Verification items for the finished model (mm, model axes). A direction names the side the tool comes from. Give positions to 0.01 mm unless a question says otherwise; leave off trailing zeros. Order: outer loops, then holes, each group sorted by start corner. A loop starts at its lowest first (then second) coordinate and runs counter-clockwise, first axis right, second up. Notation, with made-up numbers: (-9, 18) -> (41, 18) arc R14 cw to (41, 35) -> close; hole circle Ø4 at (-7, 34.5). An arc over 180 degrees is marked (long way). One line per question, with ' | ' between items. Start each with the question number.
Q1. Section check C-C on x = 52. Record the cut outline in (y, z).
Q2. Section check A-A on z = 5.25. Record the cut outline in (x, y) (1 decimal).
Q3. Go/stop test with flat-tipped pins: pin 1 (4 mm diameter, centred on x = -10.5, y = -47.5, fed in from -Z); pin 2 (1 mm diameter, centred on x = 41.5, z = 4, fed in from -Y); pin 3 (1.9 mm diameter, centred on x = -82, z = 4.5, fed in from +Y); pin 4 (2 mm diameter, centred on y = -67.5, z = 2, fed in from +X). Record where each tip stops, or that it passes through.
Q4. Material ranges on probe 1 along X at (y, z) = (52, 4.5); probe 2 along X at (y, z) = (76.5, 5.25) (3 decimals); probe 3 along Y at (x, z) = (29, 0.5), recorded low to high. Write a range as [from, to].
Q5. Section check B-B on y = 76.5. Record the cut outline in (x, z) (3 decimals), plus the area to 3 significant figures.
Q6. Mould release check, pull along Y, two halves, no side actions. Record for faces 3 (the cylindrical face through (-81.2, -79.6, 3.1)), 4 (the flat face through (9, 1, 0)): released by +Y, released by -Y, zero draft, split by the parting line, or undercut.
Q7. Access from +Z, -Z, +X, -X, +Y, -Y to the whole of each face (thin tool, end or side, straight path). Record for faces 1 (the flat face through (9, 1, 6.35)), 2 (the cylindrical face through (-79.5, 81.3, 3.1)).
from build123d import *

# Parameters (mm, degrees)
SKETCH1_R           = 123.5325
SKETCH1_R_2         = 113.71
BOSS_EXTRUDE1_DEPTH = 6.35


with BuildPart() as part:
    # Sketch1 → Boss-Extrude1 (new body)
    # profile 1 of 2: a face of its own
    with BuildSketch(Plane.XY):
        Circle(SKETCH1_R)
        Circle(SKETCH1_R_2, mode=Mode.SUBTRACT)
    # profile 2 of 2: a face of its own
    with BuildSketch(Plane.XY):
        with BuildLine():
            ThreePointArc((22.7, 12.7), (15.628932188, 15.628932188), (12.7, 22.7))
            Line((12.7, 22.7), (12.7, 112.998557955))
            ThreePointArc((12.7, 112.998557955), (0.173278497, 113.709867974), (-12.355552704, 113.036739237))
            Line((-12.355552704, 113.036739237), (-12.355552704, 22.7))
            ThreePointArc((-12.355552704, 22.7), (-15.284484892, 15.628932188), (-22.355552704, 12.7))
            Line((-22.355552704, 12.7), (-112.998557955, 12.7))
            ThreePointArc((-112.998557955, 12.7), (-113.71, 0), (-112.998557955, -12.7))
            Line((-112.998557955, -12.7), (-22.7, -12.7))
            ThreePointArc((-22.7, -12.7), (-15.628932188, -15.628932188), (-12.7, -22.7))
            Line((-12.7, -22.7), (-12.7, -112.998557955))
            ThreePointArc((-12.7, -112.998557955), (0.173337872, -113.709867883), (13.044447296, -112.959313448))
            Line((13.044447296, -112.959313448), (13.044447296, -22.7))
            ThreePointArc((13.044447296, -22.7), (15.973379485, -15.628932188), (23.044447296, -12.7))
            Line((23.044447296, -12.7), (112.998557955, -12.7))
            ThreePointArc((112.998557955, -12.7), (113.53200017, -6.359955774), (113.71, 0))
            ThreePointArc((113.71, 0), (113.53200017, 6.359955774), (112.998557955, 12.7))
            Line((112.998557955, 12.7), (22.7, 12.7))
        make_face()
    extrude(amount=BOSS_EXTRUDE1_DEPTH)


solid = part.part
Filled in:
1) outline: (-112.05, 0) -> (-101.12, 0) -> (-101.12, 6.35) -> (-112.05, 6.35) -> close; (-12.7, 0) -> (12.7, 0) -> (12.7, 6.35) -> (-12.7, 6.35) -> close; (101.12, 0) -> (112.05, 0) -> (112.05, 6.35) -> (101.12, 6.35) -> close
2) outline: circle Ø247.1 at (0, 0); hole (-113, -12.7) arc R113.7 ccw to (-12.7, -113) -> (-12.7, -22.7) arc R10 ccw to (-22.7, -12.7) -> close; hole (-113, 12.7) -> (-22.4, 12.7) arc R10 ccw to (-12.4, 22.7) -> (-12.4, 113) arc R113.7 ccw to start; hole (12.7, 22.7) arc R10 ccw to (22.7, 12.7) -> (113, 12.7) arc R113.7 ccw to (12.7, 113) -> close; hole (13, -113) arc R113.7 ccw to (113, -12.7) -> (23, -12.7) arc R10 ccw to (13, -22.7) -> close
3) pin 1: z = 0 | pin 2: y = -116.53 | pin 3: y = 93.23 | pin 4: x = 104.11
4) probe 1: [-112.05, -101.12], [-12.36, 12.7], [101.12, 112.05] | probe 2: [-96.995, -84.129], [-12.356, 12.7], [84.129, 96.995] | probe 3: [-120.08, -109.95], [-12.7, 12.7], [109.95, 120.08]
5) outline: (-96.995, 0) -> (-84.129, 0) -> (-84.129, 6.35) -> (-96.995, 6.35) -> close; (-12.356, 0) -> (12.7, 0) -> (12.7, 6.35) -> (-12.356, 6.35) -> close; (84.129, 0) -> (96.995, 0) -> (96.995, 6.35) -> (84.129, 6.35) -> close | area: 322 mm²
6) face 3: undercut | face 4: zero draft
7) face 1: +Z, +X, -X, +Y, -Y | face 2: +Z, -Z
